from build123d import *

# Parameters (mm, degrees)
CHAMFER1_SIZE = 0.254


with BuildPart() as part:
    # Sketch1 → Revolve1 (revolve)
    with BuildSketch(Plane(origin=(0, 0, 0), x_dir=(1, 0, 0), z_dir=(0, 1, 0))):
        Polygon((2.286, -10.6), (4.064, -10.6), (4.064, -16.9418), (9.4615, -16.9418), (9.4615, -15.367), (8.0264, -15.367), (8.0264, 0), (2.286, 0), align=None)
    revolve(axis=Axis((0, 0, 0), (0, 0, 1)))

    # Chamfer1
    chamfer1_edges = [part.edges().sort_by_distance(p)[0] for p in [
        (-2.286, 0, 0),
        (-8.0264, 0, 0),
        (-9.4615, 0, 15.367),
        (-9.4615, 0, 16.9418),
        (-4.064, 0, 16.9418),
        (-2.286, 0, 10.6),
    ]]
    chamfer(chamfer1_edges, length=CHAMFER1_SIZE)


solid = part.part
Can you work these out from the model? Positions are in its coordinate system, mm. A direction names the side the tool comes from. Give positions to 0.01 mm unless a question says otherwise; leave off trailing zeros. Loops run counter-clockwise (first coordinate to the right, second up) from the corner with the lowest first, then second, coordinate; pieces in that order, holes last. Notation, with made-up numbers: (18.5, -5) - (57.5, -5) arc R26 ccw to (57.5, 15) - close; hole circle Ø11 at (72.5, 57.25). An arc over 180 degrees is marked (long way). Return JSON: item names as keys, results as strings.
1. For faces 1 (the face through (-3, 8, 15.367)), 2 (the face through (2, -2, 10.6)), 3 (the face through (-0.5, -2.23, 5.37)), which set-ups out of +Z, -Z, +X, -X, +Y, -Y let a thin tool reach every point of the face, with its end or its side?
Output values:
{"face 1": "-Z", "face 2": "+Z", "face 3": "+Z, -Z"}
2. I want a section at C-C on z = 8.5. Please give me the cut outline in (x, y).
Output values:
{"outline": "circle Ø16.05 at (0, 0); hole circle Ø4.57 at (0, 0)"}
3. I want a section at A-A on y = 0. Please give me the cut outline in (x, z).
Output values:
{"outline": "(-9.46, 15.62) - (-9.21, 15.37) - (-8.03, 15.37) - (-8.03, 0.25) - (-7.77, 0) - (-2.54, 0) - (-2.29, 0.25) - (-2.29, 10.35) - (-2.54, 10.6) - (-4.06, 10.6) - (-4.06, 16.69) - (-4.32, 16.94) - (-9.21, 16.94) - (-9.46, 16.69) - close; (2.29, 0.25) - (2.54, 0) - (7.77, 0) - (8.03, 0.25) - (8.03, 15.37) - (9.21, 15.37) - (9.46, 15.62) - (9.46, 16.69) - (9.21, 16.94) - (4.32, 16.94) - (4.06, 16.69) - (4.06, 10.6) - (2.54, 10.6) - (2.29, 10.35) - close"}
4. I'm going to push flat-ended pins straight in: pin 1 Ø2 at (x, z) = (1.5, 4.5) entering from -Y; pin 2 Ø6 at (y, z) = (4, 10.5) entering from -X; pin 3 Ø1 at (x, z) = (6.5, 15) entering from +Y. Where does each tip first touch, or does it pass through?
Output values:
{"pin 1": "stops at y = -8.01", "pin 2": "stops at x = -7.96", "pin 3": "stops at y = 6.85"}
5. If I drill on line 1 (Z direction, x = -2.25, y = -2); line 2 (Z direction, x = 4.5, y = -8); line 3 (Y direction, x = 0, z = 12.75), over which ranges is the centre line in solid material (lowest first)?
Output values:
{"line 1": "z = 0 to 10.6", "line 2": "z = 15.37 to 16.94", "line 3": "y = -8.03 to -4.06, 4.06 to 8.03"}
6. We'd pull the mould along X, two halves only. Please class faces 4 (the face through (-2, 2, 0)), 5 (the face through (-0.881, -3.967, 13.687)), 6 (the face through (-5.92, 5.42, 7.7)): +X half, -X half, draft (parallel to the pull), parting line (faces both ways), or undercut.
Output values:
{"face 4": "draft", "face 5": "undercut", "face 6": "parting line"}
